The listing builds one solid part. Answer for the finished solid, in the listing's coordinates (mm). Face numbers are marked on the shaded views. Coordinates: 2 decimals unless noted, no trailing zeros. Write each loop counter-clockwise with the first axis right and the second up, starting at its lowest first coordinate (ties: lowest second). Pieces come first, ordered by that corner, then holes.
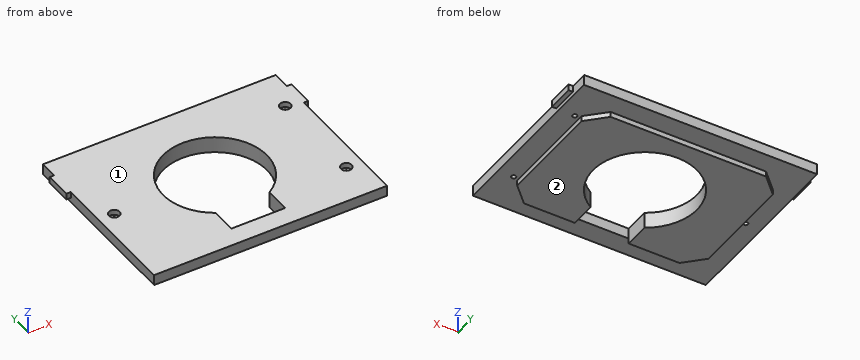
from build123d import *

# Parameters (mm, degrees)
F0_W     = 260
F0_H     = 200
F1_DEPTH = 12
F2_DEPTH = 6
F3_W     = 5
F3_H     = 30
F4_DEPTH = 7
F5_R     = 6
F5_R_2   = 2.5
F6_DEPTH = 6
F7_DEPTH = 18.001


with BuildPart() as f1:
    # F0 (on Top) → F1 (new body)
    with BuildSketch(Plane.XY):
        Rectangle(F0_W, F0_H)
        Polygon((-86.75, 78), (86.75, 78), (106.75, 58), (106.75, -58), (86.75, -78), (30, -78), (-30, -78), (-86.75, -78), (-106.75, -58), (-106.75, 58), align=None, mode=Mode.SUBTRACT)
        with BuildLine():
            Line((106.75, 58), (86.75, 78))
            Line((86.75, 78), (-86.75, 78))
            Line((-86.75, 78), (-106.75, 58))
            Line((-106.75, 58), (-106.75, -58))
            Line((-106.75, -58), (-86.75, -78))
            Line((-86.75, -78), (-30, -78))
            Line((-30, -78), (-30, -49.638695))
            ThreePointArc((-30, -49.638695), (0, 58), (30, -49.638695))
            Line((30, -49.638695), (30, -78))
            Line((30, -78), (86.75, -78))
            Line((86.75, -78), (106.75, -58))
            Line((106.75, -58), (106.75, 58))
        make_face()
    extrude(amount=F1_DEPTH)

    # F0 (on Top) → F2 (join)
    with BuildSketch(Plane.XY):
        with BuildLine():
            Line((106.75, 58), (86.75, 78))
            Line((86.75, 78), (-86.75, 78))
            Line((-86.75, 78), (-106.75, 58))
            Line((-106.75, 58), (-106.75, -58))
            Line((-106.75, -58), (-86.75, -78))
            Line((-86.75, -78), (-30, -78))
            Line((-30, -78), (-30, -49.638695))
            ThreePointArc((-30, -49.638695), (0, 58), (30, -49.638695))
            Line((30, -49.638695), (30, -78))
            Line((30, -78), (86.75, -78))
            Line((86.75, -78), (106.75, -58))
            Line((106.75, -58), (106.75, 58))
        make_face()
    extrude(amount=-F2_DEPTH)

    # F3 (on face) → F4 (join)
    with BuildSketch(Plane.XY.offset(12)):
        with Locations((-132.5, 65)):
            Rectangle(F3_W, F3_H)
        with Locations((132.5, 65)):
            Rectangle(F3_W, F3_H)
    extrude(amount=-F4_DEPTH)

    # F5 (on face) → F6 (cut)
    with BuildSketch(Plane.XY.offset(12)):
        with Locations((-112.5, 0)):
            Circle(F5_R)
        with Locations((-112.5, 0)):
            Circle(F5_R_2, mode=Mode.SUBTRACT)
        with Locations((-112.5, 0)):
            Circle(F5_R_2)
        with Locations((112.5, 55)):
            Circle(F5_R)
        with Locations((112.5, 55)):
            Circle(F5_R_2, mode=Mode.SUBTRACT)
        with Locations((112.5, 55)):
            Circle(F5_R_2)
        with Locations((112.5, -55)):
            Circle(F5_R_2)
        with Locations((112.5, -55)):
            Circle(F5_R)
        with Locations((112.5, -55)):
            Circle(F5_R_2, mode=Mode.SUBTRACT)
    extrude(amount=-F6_DEPTH, mode=Mode.SUBTRACT)

    # F5 (on face) → F7 (cut, through all)
    with BuildSketch(Plane.XY.offset(12)):
        with Locations((-112.5, 0)):
            Circle(F5_R_2)
        with Locations((112.5, 55)):
            Circle(F5_R_2)
        with Locations((112.5, -55)):
            Circle(F5_R_2)
    extrude(amount=-F7_DEPTH, mode=Mode.SUBTRACT)


solid = f1.part
Q1. Determine the mould class of the marked faces 1 and 2 for opening direction Z: released by +Z, released by -Z, zero draft, split by the parting line, or undercut.
Answers below:
face 1: released by +Z
face 2: released by -Z
Q2. Find the intervals of material crossed by probe 1 along Y at (x, z) = (112.5, 7.65); probe 2 along Y at (x, z) = (112.5, 1.2); probe 3 along X at (y, z) = (-50.5, 9), in increasing order.
Answers below:
probe 1: y = -100 to -61, -49 to 49, 61 to 100
probe 2: y = -100 to -57.5, -52.5 to 52.5, 57.5 to 100
probe 3: x = -130 to -30, 30 to 108.53, 116.47 to 130
Q3. The part is cut by section B-B, the plane y = -12. Write down the section's boundary in (x, z), then the cut area to 3 significant figures.
Answers below:
outline: (-130, 0) - (-106.75, 0) - (-106.75, -6) - (-56.75, -6) - (-56.75, 12) - (-130, 12) - close; (56.75, -6) - (106.75, -6) - (106.75, 0) - (130, 0) - (130, 12) - (56.75, 12) - close
area: 2,360 mm2
Q4. The part is cut by section C-C, the plane y = -44. Write down the section's boundary in (x, z), then the cut area to 3 significant figures.
Answers below:
outline: (-130, 0) - (-106.75, 0) - (-106.75, -6) - (-37.79, -6) - (-37.79, 12) - (-130, 12) - close; (37.79, -6) - (106.75, -6) - (106.75, 0) - (130, 0) - (130, 12) - (37.79, 12) - close
area: 3,040 mm2
Q5. The part is cut by section A-A, the plane x = 0. Write down the section's boundary in (y, z).
Answers below:
outline: (-100, 0) - (-78, 0) - (-78, 12) - (-100, 12) - close; (58, -6) - (78, -6) - (78, 0) - (100, 0) - (100, 12) - (58, 12) - close
Q6. Given pin 1 (6 mm diameter, centred on x = 115, y = 53.5, fed in from +Z); pin 2 (9.5 mm diameter, centred on y = -22, z = 8.5, fed in from -X); pin 3 (1.8 mm diameter, centred on y = -11, z = -2.5, fed in from -X), each flat-ended and moving along its own axis, determine where each tip first touches the part or whether it passes through.
Answers below:
pin 1: stops at z = 6
pin 2: stops at x = -130
pin 3: stops at x = -106.75
